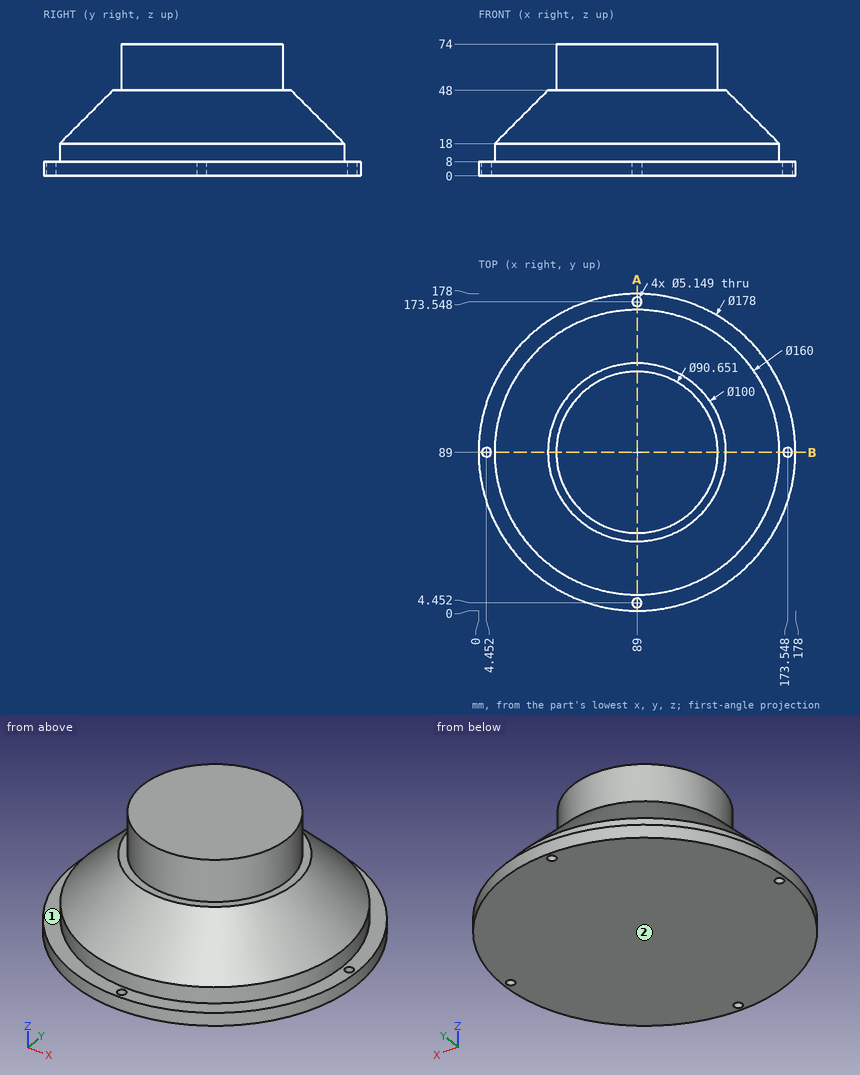
The figure shows three views and two pictorial views of one solid part (mm, origin at its lowest corner). Answer the questions. A direction names the side the tool comes from. Round coordinates to 2 decimals unless told otherwise and drop trailing zeros. Order: outer loops, then holes, each group sorted by start corner. A loop starts at its lowest first (then second) coordinate and runs counter-clockwise, first axis right, second up. Notation, with made-up numbers: (7, 35.5) -> (36, 35.5) arc R17 cw to (36, 52.5) -> close; hole circle Ø11 at (-30.75, 26.25). An arc over 180 degrees is marked (long way). Put each result on its own line as item: value.
Q1. Consider line 1 along Y through (x, z) = (89, 5); line 2 along Z through (x, y) = (114, 9.5); line 3 along Y through (x, z) = (54.5, 52.5) (1 decimal). Determine where each line is inside the solid, lowest interval first.
Results list:
line 1: 0 to 1.88, 7.03 to 170.97, 176.12 to 178
line 2: 0 to 8
line 3: 59.6 to 118.4
Q2. Each of these flat-tipped pins is pushed along its axis until it touches: P1, Ø8, axis at x = 97.5, z = 53, coming from the +Y side; P2, Ø10, axis at x = 92.5, y = 78.5, coming from the -Z side; P3, Ø6.5, axis at x = 173.55, y = 89, coming from the +Z side; P4, Ø4, axis at y = 43.5, z = 28.5, coming from the +X side (1 decimal). Where does it stop, or does it pass through?
Results list:
P1: y = 134.1
P2: z = 0
P3: z = 8
P4: x = 144.6
Q3. Which of the six approach directions +Z, -Z, +X, -X, +Y, -Y give full straight-line access (tool end or side, diameter ignored) to the marked faces 1 and 2?
Results list:
face 1: +Z
face 2: -Z, +X, -X, +Y, -Y
Q4. Section A-A, the plane x = 89 is taken. Write down the section's boundary in (y, z) (1 decimal), and give its area (3 significant figures).
Results list:
outline: (0, 0) -> (1.9, 0) -> (1.9, 8) -> (0, 8) -> close; (7, 0) -> (171, 0) -> (171, 8) -> (169, 8) -> (169, 18) -> (139, 48) -> (134.3, 48) -> (134.3, 74) -> (43.7, 74) -> (43.7, 48) -> (39, 48) -> (9, 18) -> (9, 8) -> (7, 8) -> close; (176.1, 0) -> (178, 0) -> (178, 8) -> (176.1, 8) -> close
area: 9,200 mm^2
